The listing builds one solid part. Answer for the finished solid, in the listing's coordinates (mm). Face numbers are marked on the shaded views. A direction names the side the tool comes from. Round coordinates to 2 decimals unless told otherwise and drop trailing zeros. Write each loop counter-clockwise with the first axis right and the second up, starting at its lowest first coordinate (ties: lowest second). Pieces come first, ordered by that corner, then holes. Notation, with made-up numbers: (70.25, -26) -> (89.25, -26) arc R12 cw to (89.25, -22) -> close; hole circle Ø2 at (64.25, 14). An arc over 180 degrees is marked (long way). Write each question's results on one line, items separated by ' | '. Start each with the question number.
```python
from build123d import *

# Parameters (mm, degrees)
BOSS_EXTRUDE1_START       = 4.524999897
BOSS_EXTRUDE1_2_OUTLINE_R = 5.225
BOSS_EXTRUDE1_2_DEPTH     = 30.925000207
SKETCH2_R                 = 8.5
BOSS_EXTRUDE2_DEPTH       = 2.5
SKETCH3_R                 = 7.8
SKETCH3_R_2               = 6
CUT_EXTRUDE1_DEPTH        = 1.15
SKETCH4_R                 = 5.225
BOSS_EXTRUDE3_DEPTH       = 4.5
CHAMFER1_SIZE             = 0.05
CHAMFER2_SIZE             = 0.799999999
CHAMFER2_SIZE2            = 0.800000001
FILLET1_R                 = 0.2


with BuildPart() as part:
    # Boss-Extrude1: read off the stored shape, not the designer's step
    # Boss-Extrude1 outline → Boss-Extrude1 (revolve)
    with BuildSketch(Plane.XZ):
        Polygon((5.225, 4.499999999), (5.225, 35.475000001), (5.2, 35.500000001), (5.2, 36.5), (0, 36.5), (0, 4.499999999), align=None)
    revolve(axis=Axis((0, 0, 0), (0, 0, 1)))

    # Boss-Extrude1 2 outline → Boss-Extrude1 2 (add)
    with BuildSketch(Plane.XY.offset(BOSS_EXTRUDE1_START)):
        with BuildLine():
            ThreePointArc((5.25, 2.904737509), (0, 6), (-5.25, 2.904737509))
            Line((-5.25, 2.904737509), (-5.25, -2.90473751))
            ThreePointArc((-5.25, -2.90473751), (0, -6), (5.25, -2.90473751))
            Line((5.25, -2.90473751), (5.25, 2.904737509))
        make_face()
        Circle(BOSS_EXTRUDE1_2_OUTLINE_R, mode=Mode.SUBTRACT)
    extrude(amount=BOSS_EXTRUDE1_2_DEPTH)

    # Boss-Extrude1 3 outline → Boss-Extrude1 3 (revolve, cut)
    with BuildSketch(Plane.XZ):
        Polygon((6, 5.275000001), (5.249999898, 4.524999897), (6, 4.524999897), align=None)
        Polygon((5.249999897, 35.450000104), (6, 34.699999999), (6, 35.450000104), align=None)
    revolve(axis=Axis((0, 0, 0), (0, 0, 1)), mode=Mode.SUBTRACT)

    # Boss-Extrude1 4 outline → Boss-Extrude1 4 (revolve)
    with BuildSketch(Plane.XZ):
        Polygon((5.225, 4.524999897), (5.225, 4.499999999), (5.249999898, 4.524999897), align=None)
        Polygon((5.225, 35.450000104), (5.249999897, 35.450000104), (5.225, 35.475000001), align=None)
    revolve(axis=Axis((0, 0, 0), (0, 0, 1)))

    # Sketch2 → Boss-Extrude2 (add)
    with BuildSketch(Plane(origin=(0, 0, 36.5), x_dir=(-1, 0, 0), z_dir=(0, 0, -1))):
        with Locations(Location((0, 0, 0), (0, 0, 180))):
            Circle(SKETCH2_R)
    extrude(amount=-BOSS_EXTRUDE2_DEPTH)

    # Sketch3 → Cut-Extrude1 (cut)
    with BuildSketch(Plane(origin=(0, 0, 36.5), x_dir=(-1, 0, 0), z_dir=(0, 0, -1))):
        with Locations(Location((0, 0, 0), (0, 0, 180))):
            Circle(SKETCH3_R)
        with Locations(Location((0, 0, 0), (0, 0, 180))):
            Circle(SKETCH3_R_2, mode=Mode.SUBTRACT)
    extrude(amount=-CUT_EXTRUDE1_DEPTH, mode=Mode.SUBTRACT)

    # Sketch4 → Boss-Extrude3 (add)
    with BuildSketch(Plane(origin=(0, 0, 4.5), x_dir=(-1, 0, 0), z_dir=(0, 0, -1))):
        Circle(SKETCH4_R)
    extrude(amount=BOSS_EXTRUDE3_DEPTH)

    # Chamfer1
    chamfer1_edges = [part.edges().sort_by_distance(p)[0] for p in [
        (5.225, 0, 0),
    ]]
    chamfer(chamfer1_edges, length=CHAMFER1_SIZE)

    # Chamfer2
    chamfer2_edges = [part.edges().sort_by_distance(p)[0] for p in [
        (-8.5, 0, 39),
    ]]
    chamfer2_side = [part.faces().sort_by_distance(p)[0] for p in [
        (-8.5, 0, 37.75),
    ]]
    chamfer(chamfer2_edges, length=CHAMFER2_SIZE, length2=CHAMFER2_SIZE2, reference=chamfer2_side[0])

    # Fillet1
    fillet1_edges = [part.edges().sort_by_distance(p)[0] for p in [
        (-7.8, 0, 37.65),
        (-6, 0, 37.65),
    ]]
    fillet(fillet1_edges, radius=FILLET1_R)


solid = part.part
```
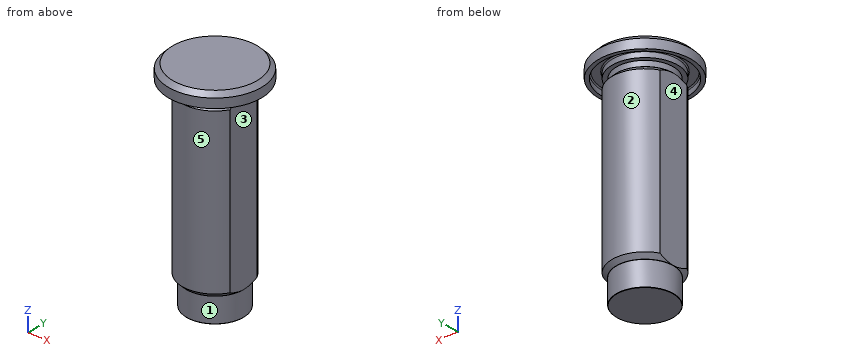
Q1. Find the intervals of material crossed by line 1 (Y direction, x = 0, z = 37.2); line 2 (Y direction, x = 4.75, z = 37.5); line 3 (Z direction, x = -6.75, y = -1.5), in increasing order.
Q2. For the marked faces 1, 2, 3, 4 and 5, determine the directions among +Z, -Z, +X, -X, +Y, -Y from which every point of the face is accessible in a straight line to the end or side of a thin tool.
Q3. Each of these flat-tipped pins is pushed along its axis until it touches: pin 1 (8 mm diameter, centred on x = 4, z = 25.5, fed in from -Y); pin 2 (3.5 mm diameter, centred on x = -1, y = 2.5, fed in from -Z); pin 3 (3 mm diameter, centred on x = -6.5, z = 25.5, fed in from +Y); pin 4 (4.5 mm diameter, centred on y = 1, z = 19.5, fed in from -X). Where does it stop, or does it pass through?
Q4. The part is cut by section A-A, the plane z = 14. Write down the section's boundary in (x, y).
Answers follow:
1) line 1: -8.5 to -7.8, -6 to 6, 7.8 to 8.5 | line 2: -7.05 to -6.18, -3.68 to 3.68, 6.18 to 7.05 | line 3: 37.65 to 39
2) face 1: -Z | face 2: -Z, +Y | face 3: -Z, +X, +Y, -Y | face 4: -Z, -X, +Y, -Y | face 5: -Z, -Y
3) pin 1: y = -6 | pin 2: z = 0 | pin 3: y = 3.32 | pin 4: x = -5.25
4) outline: (-5.25, -2.9) arc R6 ccw to (5.25, -2.9) -> (5.25, 2.9) arc R6 ccw to (-5.25, 2.9) -> close
